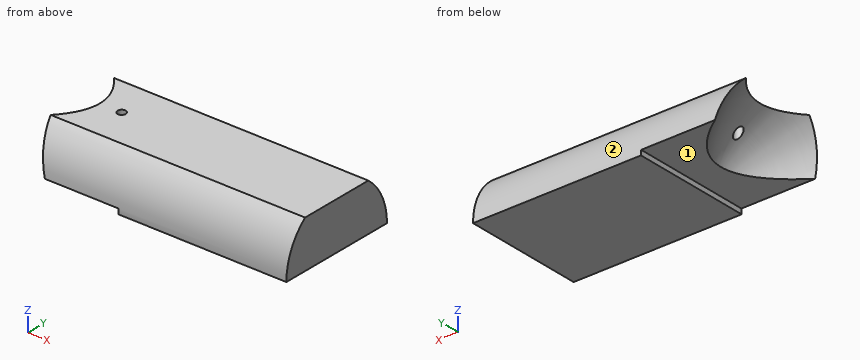
from build123d import *

# Parameters (mm, degrees)
CYLINDER001_R     = 2.185
CYLINDER001_DEPTH = 9.314408
BOX_W             = 9.314408
BOX_H             = 4.37
BOX_DEPTH         = 0.935
BOX001_W          = 3.259408
BOX001_H          = 4.37
BOX001_DEPTH      = 0.63
BOX002_W          = 9.314408
BOX002_H          = 4.37
BOX002_DEPTH      = 0.55
CYLINDER_R        = 0.15
CYLINDER_DEPTH    = 2.185
REVOLUTION_ANGLE  = 180


with BuildPart() as volumelimit:
    # Cylinder001 → Cylinder001 (new body)
    with BuildSketch(Plane(origin=(-1.564408, 0, 0), x_dir=(0, 0, -1), z_dir=(1, 0, 0))):
        Circle(CYLINDER001_R)
    extrude(amount=CYLINDER001_DEPTH)


with BuildPart() as upperedgecuttingtool:
    # Box → Box (new body)
    with BuildSketch(Plane(origin=(-1.564408, -2.185, 1.7), x_dir=(1, 0, 0), z_dir=(0, 0, 1))):
        with Locations((4.657204, 2.185)):
            Rectangle(BOX_W, BOX_H)
    extrude(amount=BOX_DEPTH)


with BuildPart() as lowerstepcuttingtool:
    # Box001 → Box001 (new body)
    with BuildSketch(Plane(origin=(-1.564408, -2.185, -0.45), x_dir=(1, 0, 0), z_dir=(0, 0, 1))):
        with Locations((1.629704, 2.185)):
            Rectangle(BOX001_W, BOX001_H)
    extrude(amount=BOX001_DEPTH)


with BuildPart() as obj1:
    # Box002 → Box002 (new body)
    with BuildSketch(Plane(origin=(-1.564408, -2.185, -0.55), x_dir=(1, 0, 0), z_dir=(0, 0, 1))):
        with Locations((4.657204, 2.185)):
            Rectangle(BOX002_W, BOX002_H)
    extrude(amount=BOX002_DEPTH)


with BuildPart() as cuttingtools:
    # Cylinder → Cylinder (new body)
    with BuildSketch(Plane.XY):
        Circle(CYLINDER_R)
    extrude(amount=CYLINDER_DEPTH)

    # Fusion: union UpperEdgeCuttingTool, LowerStepCuttingTool, obj1
    add(upperedgecuttingtool.part)
    add(lowerstepcuttingtool.part)
    add(obj1.part)


with BuildPart() as mirrorwithoutmount:
    # Sketch → Revolution (revolve)
    with BuildSketch(Plane.XY):
        with BuildLine():
            Line((0.75, 0), (7.75, 0))
            Line((7.75, 0), (7.75, 2.635))
            Line((7.75, 2.635), (-1.564408, 2.635))
            add(Edge.make_bspline(
                [(-1.564408, 2.635), (0.75, 1.3175), (0.75, 0)],
                knots=[-2.635, -2.635, -2.635, 0, 0, 0], degree=2))
        make_face()
    revolve(axis=Axis((0, 0, 0), (1, 0, 0)), revolution_arc=REVOLUTION_ANGLE)


with BuildPart() as mirrorwithoutmount_1:
    # Body001 placement: moved
    add(mirrorwithoutmount.part.moved(Location((0, 0, -0.45))))

    # Cut: cut CuttingTools
    add(cuttingtools.part, mode=Mode.SUBTRACT)

    # Common: intersect VolumeLimit
    add(volumelimit.part, mode=Mode.INTERSECT)


solid = mirrorwithoutmount_1.part
Can you work these out from the model? Positions are in its coordinate system, mm. Face numbers are marked on the shaded views. A direction names the side the tool comes from. Coordinates: 2 decimals unless noted, no trailing zeros. Loops run counter-clockwise (first coordinate to the right, second up) from the corner with the lowest first, then second, coordinate; pieces in that order, holes last. Notation, with made-up numbers: (64.5, -39.5) - (82.5, -39.5) arc R24 ccw to (82.5, -28.5) - close; hole circle Ø11 at (-33.75, 70). An arc over 180 degrees is marked (long way). Answer as a JSON object with one key per item and string values. Group by question number.
Item 1: If we section it at A-A (x = 1.25): List the corners of the cut face in (y, z) for me (3 decimals), plus the area to 3 significant figures.
Item 2: On a 3-axis mill with a long thin cutter (end or side, diameter ignored), from which of +Z, -Z, +X, -X, +Y, -Y can I reach the whole of each face in a straight line? I mean the marked faces 1 and 2. Say none if no direction works.
Item 3: If we section it at B-B (x = 4.5): List the corners of the cut face in (y, z) for me (3 decimals), plus the area to 3 significant figures.
Item 4: For pin 1 (1.5 mm diameter, centred on x = 4.5, y = 1.5, fed in from -Z), with a flat end and sliding along its axis, tell me the tip position at first contact or that it passes through.
Item 5: If I drill on L1, parallel to Z at x = 2.5, y = -1.7; L2, parallel to X at y = 0, z = 1.4; L3, parallel to Y at x = 0, z = 1.15, over which ranges is the centre line in solid material (lowest first)? Write a range as from..to.
Returned:
{
 "1": {"outline": "(-2.178, 0.18) - (2.178, 0.18) arc R2.185 ccw to (1.373, 1.7) - (-1.373, 1.7) arc R2.185 ccw to start", "area": "5.80 mm²"},
 "2": {"face 1": "-Z, -X, +Y, -Y", "face 2": "+Z, +X, -X, +Y"},
 "3": {"outline": "(-2.185, 0) - (2.185, 0) arc R2.185 ccw to (1.373, 1.7) - (-1.373, 1.7) arc R2.185 ccw to start", "area": "6.59 mm²"},
 "4": {"pin 1": "stops at z = 0"},
 "5": {"L1": "z = 0..1.37", "L2": "x = -0.39..-0.15, 0.15..7.75", "L3": "y = -1.86..-0.15, 0.15..1.86"}
}
